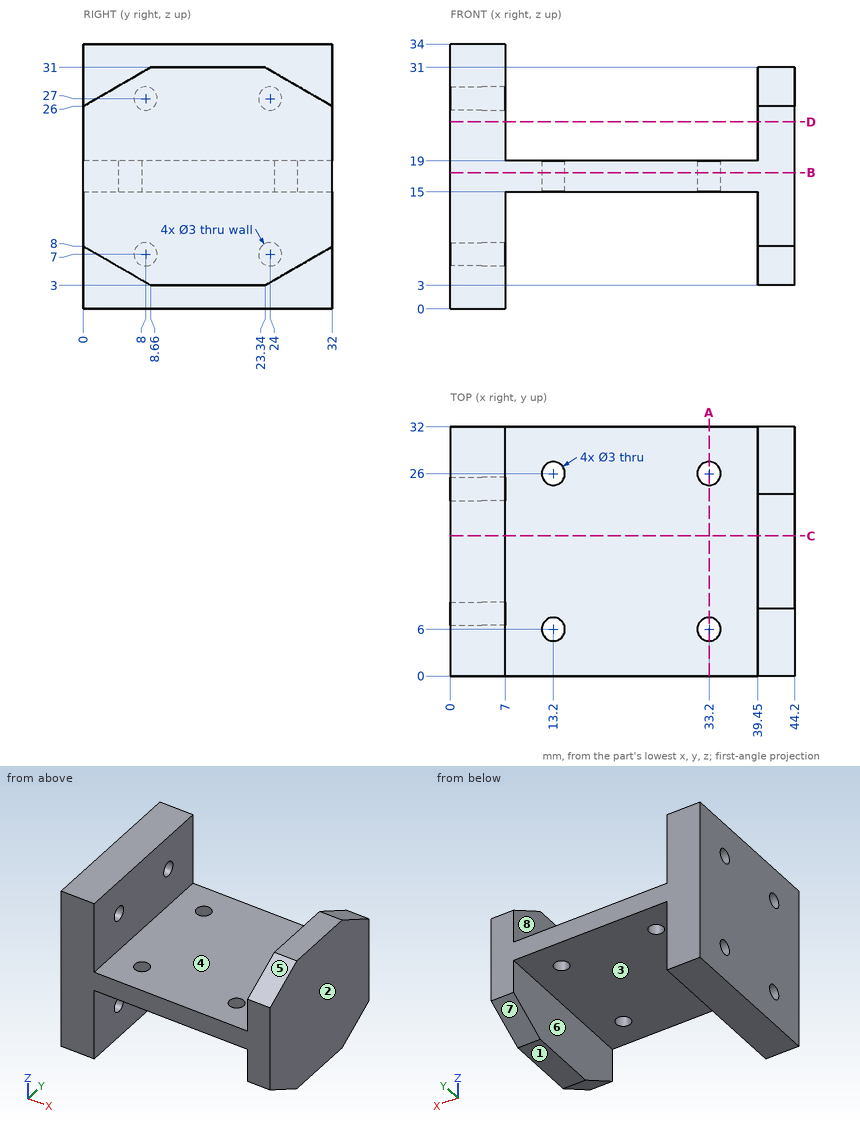
Can you work these out from the drawing? Everything is in mm from the part's minimum corner. A direction names the side the tool comes from. Coordinates: 2 decimals unless noted, no trailing zeros. Write each loop counter-clockwise with the first axis right and the second up, starting at its lowest first coordinate (ties: lowest second). Pieces come first, ordered by that corner, then holes. Notation, with made-up numbers: (-33.75, 67) - (-14.75, 67) arc R12 cw to (-14.75, 88) - close; hole circle Ø8 at (0.25, 14.25). An arc over 180 degrees is marked (long way). One line per item, written item: value.
1) On a 3-axis mill with a long thin cutter (end or side, diameter ignored), from which of +Z, -Z, +X, -X, +Y, -Y can I reach the whole of each face in a straight line? I mean the marked faces 5, 6, 7 and 8. Say none if no direction works.
Model answer:
face 5: +Z, +X, -Y
face 6: -Z, +Y, -Y
face 7: -Z, +X, +Y
face 8: +Z, +Y, -Y
2) I need wall thicknesses on line 1 along Y through (x, z) = (1.05, 27); line 2 along Y through (x, z) = (33.2, 18.05); line 3 along X through (y, z) = (14, 7). Which ranges of each line are inside material? Lowest first, please.
Model answer:
line 1: y = 0 to 6.5, 9.5 to 22.5, 25.5 to 32
line 2: y = 0 to 4.5, 7.5 to 24.5, 27.5 to 32
line 3: x = 0 to 7, 39.45 to 44.2
3) Suppose I cut it at B-B on z = 17.5. Write out the boundary of the cut face in (x, y), and give its area (3 significant figures).
Model answer:
outline: (0, 0) - (44.2, 0) - (44.2, 32) - (0, 32) - close; hole circle Ø3 at (13.2, 6); hole circle Ø3 at (13.2, 26); hole circle Ø3 at (33.2, 6); hole circle Ø3 at (33.2, 26)
area: 1,390 mm²
4) Suppose I cut it at A-A on x = 33.2. Write out the boundary of the cut face in (y, z).
Model answer:
outline: (0, 15) - (4.5, 15) - (4.5, 19) - (0, 19) - close; (7.5, 15) - (24.5, 15) - (24.5, 19) - (7.5, 19) - close; (27.5, 15) - (32, 15) - (32, 19) - (27.5, 19) - close
5) We'd pull the mould along X, two halves only. Please class the marked faces 1, 2, 3 and 4: pulls with the +X half, pulls with the -X half, needs draft (parallel to the pull), parting line crosses it, or undercut.
Model answer:
face 1: needs draft
face 2: pulls with the +X half
face 3: undercut
face 4: undercut
6) Suppose I cut it at D-D on z = 24. Write out the boundary of the cut face in (x, y).
Model answer:
outline: (0, 0) - (7, 0) - (7, 32) - (0, 32) - close; (39.45, 0) - (44.2, 0) - (44.2, 32) - (39.45, 32) - close
7) Suppose I cut it at C-C on y = 18. Write out the boundary of the cut face in (x, z), and give its area (3 significant figures).
Model answer:
outline: (0, 0) - (7, 0) - (7, 15) - (39.45, 15) - (39.45, 3) - (44.2, 3) - (44.2, 31) - (39.45, 31) - (39.45, 19) - (7, 19) - (7, 34) - (0, 34) - close
area: 501 mm²
8) I'm going to push flat-ended pins straight in: P1, Ø4, axis at x = 33.5, z = 22.5, coming from the -Y side; P2, Ø4, axis at x = 41, y = 14, coming from the -Z side; P3, Ø2.5, axis at x = 43, y = 14.5, coming from the +Z side; P4, Ø4, axis at x = 18, y = 14, coming from the +Z side. Where does each tip first touch, or does it pass through?
Model answer:
P1: passes through
P2: stops at z = 3
P3: stops at z = 31
P4: stops at z = 19
